```python
from build123d import *

# Parameters (mm, degrees)
ESBO_O4_R                = 3.5
RESSALTO_EXTRUS_O1_DEPTH = 3


with BuildPart() as part:
    # Esboço4 → Ressalto-extrusão1 (new body)
    with BuildSketch(Plane(origin=(0, 0, 0), x_dir=(1, 0, 0), z_dir=(0, 1, 0))):
        Polygon((19.1, 6.75), (16.6, 6.75), (16.6, 8), (14.1, 8), (14.1, 11), (16.6, 11), (16.6, 12.25), (19.1, 12.25), (19.1, 11), (23.1, 11), (23.1, 18), (-0.5, 18), (-22.5, 18), (-22.5, 11), (-18.5, 11), (-18.5, 12.25), (-16, 12.25), (-16, 11), (-13.5, 11), (-13.5, 8), (-16, 8), (-16, 6.75), (-18.5, 6.75), (-18.5, 8), (-22.5, 8), (-22.5, 5), (-25.5, 5), (-25.5, -5), (-22.5, -5), (-22.5, -8), (-18.5, -8), (-18.5, -6.75), (-16, -6.75), (-16, -8), (-13.5, -8), (-13.5, -11), (-16, -11), (-16, -12.25), (-18.5, -12.25), (-18.5, -11), (-22.5, -11), (-22.5, -18), (-0.5, -18), (23.1, -18), (23.1, -11), (19.1, -11), (19.1, -12.25), (16.6, -12.25), (16.6, -11), (14.1, -11), (14.1, -8), (16.6, -8), (16.6, -6.75), (19.1, -6.75), (19.1, -8), (23.1, -8), (23.1, -5), (26.1, -5), (26.1, 5), (23.1, 5), (23.1, 8), (19.1, 8), align=None)
        with Locations(Location((0.3, 0, 0), (0, 0, 270))):
            Circle(ESBO_O4_R, mode=Mode.SUBTRACT)
        Polygon((0.3, -15), (-0.2, -15), (-0.2, -9), (0.8, -9), (0.8, -15), align=None, mode=Mode.SUBTRACT)
        Polygon((0.8, 15), (0.3, 15), (-0.2, 15), (-0.2, 9), (0.8, 9), align=None, mode=Mode.SUBTRACT)
    extrude(amount=RESSALTO_EXTRUS_O1_DEPTH)


solid = part.part
```
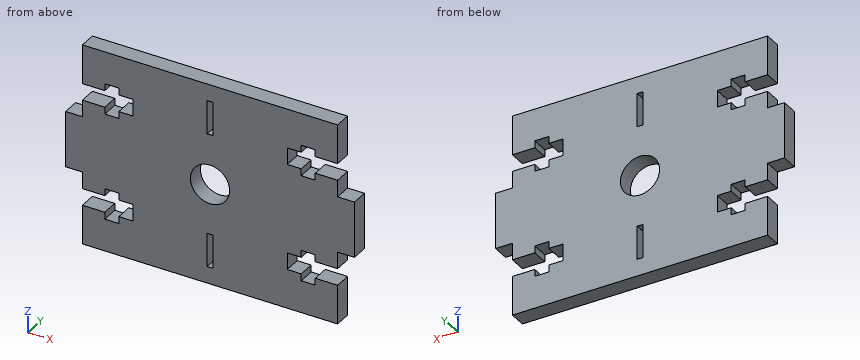
Geometry: final body of the model. Coordinates: model frame, mm. Round coordinates to 2 decimals unless told otherwise and drop trailing zeros. Write each loop counter-clockwise with the first axis right and the second up, starting at its lowest first coordinate (ties: lowest second). Pieces come first, ordered by that corner, then holes. Notation, with made-up numbers: M -12,56.25 L 1,56.25 A28 cw 1,80.25 Z; hole C 89.25,75.25 d10. An arc over 180 degrees is marked long. Answer in a Markdown table with one row per item. Add a question column.
(1) Contact query for flat-ended pins moving along their axis: pin 1 (1 mm diameter, centred on y = 2, z = 11.5, fed in from -X); pin 2 (1.5 mm diameter, centred on x = -0.5, z = -0.5, fed in from -Y); pin 3 (1.4 mm diameter, centred on y = 1.5, z = 7, fed in from +X). Output: stop coordinate, or through.
(2) Ray query, L1, parallel to X at y = 1.9, z = -11.5; L2, parallel to Z at x = 20.5, y = 2.15; L3, parallel to X at y = 2.8, z = -7. Return the intervals inside material, ascending.
(3) Cut plane A-A, the plane x = 16. Return the cut outline in (y, z).
(4) Cut plane B-B, the plane z = -10. Return the cut outline in (x, y), then the cut area to 3 significant figures.
(5) Cut plane D-D, the plane x = -17.5. Return the cut outline in (y, z).
(6) Cut plane C-C, the plane y = 1.8. Give the number of separate pieces and of enclosed holes in the cut face, then the cut area to 3 significant figures.
Established:
| question | item | result |
|---|---|---|
| 1 | pin 1 | x = -22.5 |
| 1 | pin 2 | through |
| 1 | pin 3 | x = 23.1 |
| 2 | L1 | -22.5 to -18.5, -16 to -0.2, 0.8 to 16.6, 19.1 to 23.1 |
| 2 | L2 | -18 to -11, -8 to 8, 11 to 18 |
| 2 | L3 | -22.5 to -18.5, -16 to 16.6, 19.1 to 23.1 |
| 3 | outline | M 0,-18 L 3,-18 L 3,-11 L 0,-11 Z; M 0,-8 L 3,-8 L 3,8 L 0,8 Z; M 0,11 L 3,11 L 3,18 L 0,18 Z |
| 4 | outline | M -13.5,0 L -0.2,0 L -0.2,3 L -13.5,3 Z; M 0.8,0 L 14.1,0 L 14.1,3 L 0.8,3 Z |
| 4 | area | 79.8 mm² |
| 5 | outline | M 0,-18 L 3,-18 L 3,-12.25 L 0,-12.25 Z; M 0,-6.75 L 3,-6.75 L 3,6.75 L 0,6.75 Z; M 0,12.25 L 3,12.25 L 3,18 L 0,18 Z |
| 6 | separate pieces | 1 |
| 6 | enclosed holes | 3 |
| 6 | area | 1,520 mm² |
